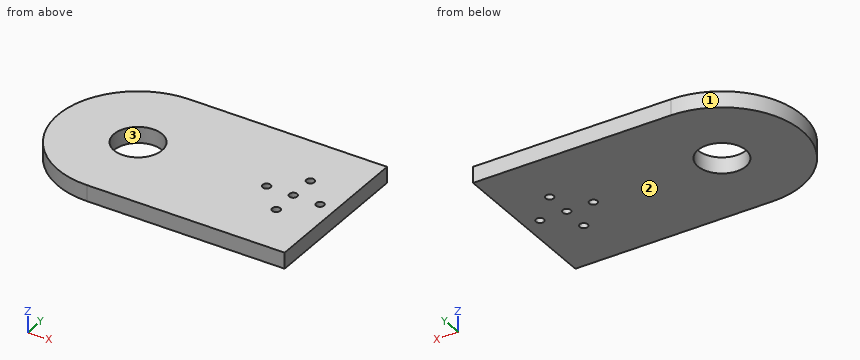
from build123d import *

# Parameters (mm, degrees)
SALIENTE_EXTRUIR1_DEPTH = 6
CROQUIS2_R              = 1.5
CORTAR_EXTRUIR1_DEPTH   = 74.654599313
CROQUIS3_R              = 9
CORTAR_EXTRUIR2_DEPTH   = 74.654599313


with BuildPart() as part:
    # Croquis1 → Saliente-Extruir1 (new body)
    with BuildSketch(Plane.XY):
        with BuildLine():
            Line((-37, 30), (37, 30))
            Line((37, 30), (37, -30))
            Line((37, -30), (-37, -30))
            ThreePointArc((-37, -30), (-67, 0), (-37, 30))
        make_face()
    extrude(amount=SALIENTE_EXTRUIR1_DEPTH)

    # Croquis2 → Cortar-Extruir1 (cut, through all)
    with BuildSketch(Plane.XY.offset(6)):
        with Locations((21.0941, -10)):
            Circle(CROQUIS2_R)
        with Locations((21.0941, 0)):
            Circle(CROQUIS2_R)
        with Locations((21.0941, 10)):
            Circle(CROQUIS2_R)
        with Locations((31.0941, 0)):
            Circle(CROQUIS2_R)
        with Locations((11.0941, 0)):
            Circle(CROQUIS2_R)
    extrude(amount=-CORTAR_EXTRUIR1_DEPTH, mode=Mode.SUBTRACT)

    # Croquis3 → Cortar-Extruir2 (cut, through all)
    with BuildSketch(Plane.XY.offset(6)):
        with Locations((-37, 0)):
            Circle(CROQUIS3_R)
    extrude(amount=-CORTAR_EXTRUIR2_DEPTH, mode=Mode.SUBTRACT)


solid = part.part
CAD build for the part. Positions are in the model's coordinates, mm. Face numbers are marked on the shaded views. Coordinates: 2 decimals unless noted, no trailing zeros. Write each loop counter-clockwise with the first axis right and the second up, starting at its lowest first coordinate (ties: lowest second). Pieces come first, ordered by that corner, then holes. Notation, with made-up numbers: M 53,58.25 L 94,58.25 A19 ccw 94,78.25 Z; hole C -23,-38 d11. An arc over 180 degrees is marked long. Return JSON: item names as keys, results as strings.
Item 1: Slice it at C-C, the plane y = 6.5. Write the cut outline in (x, z).
Findings below:
{"outline": "M -66.29,0 L -43.22,0 L -43.22,6 L -66.29,6 Z; M -30.78,0 L 37,0 L 37,6 L -30.78,6 Z"}
Item 2: Slice it at A-A, the plane y = 0. Write the cut outline in (x, z), and give its area (3 significant figures).
Findings below:
{"outline": "M -67,0 L -46,0 L -46,6 L -67,6 Z; M -28,0 L 9.59,0 L 9.59,6 L -28,6 Z; M 12.59,0 L 19.59,0 L 19.59,6 L 12.59,6 Z; M 22.59,0 L 29.59,0 L 29.59,6 L 22.59,6 Z; M 32.59,0 L 37,0 L 37,6 L 32.59,6 Z", "area": "462 mm2"}
Item 3: Slice it at B-B, the plane z = 1.4. Write the cut outline in (x, y).
Findings below:
{"outline": "M -37,-30 L 37,-30 L 37,30 L -37,30 A30 ccw Z; hole C -37,0 d18; hole C 11.09,0 d3; hole C 21.09,-10 d3; hole C 21.09,0 d3; hole C 21.09,10 d3; hole C 31.09,0 d3"}
Item 4: Two-plate mould, pull along X, no slides. Class the marked faces 1, 2 and 3: +X half, -X half, draft (parallel to the pull), parting line (faces both ways), or undercut.
Findings below:
{"face 1": "-X half", "face 2": "draft", "face 3": "undercut"}
Item 5: Slice it at D-D, the plane x = 11.5. Write the cut outline in (y, z).
Findings below:
{"outline": "M -30,0 L -1.44,0 L -1.44,6 L -30,6 Z; M 1.44,0 L 30,0 L 30,6 L 1.44,6 Z"}
Item 6: Probe line 1 (Y direction, x = -37.5, z = 1.65); line 2 (X direction, y = 5, z = 2.45); line 3 (X direction, y = 24, z = 2.9). List the from-to ranges inside material, lowest first. Write a range as from..to.
Findings below:
{"line 1": "y = -30..-8.99, 8.99..30", "line 2": "x = -66.58..-44.48, -29.52..37", "line 3": "x = -55..37"}
